Read the model definition and answer for the solid it produces. Units are mm, in the model's axes. A direction names the side the tool comes from. Coordinates: 2 decimals unless noted, no trailing zeros. Loops run counter-clockwise (first coordinate to the right, second up) from the corner with the lowest first, then second, coordinate; pieces in that order, holes last. Notation, with made-up numbers: M 75,34 L 123,34 A28 cw 123,56 Z; hole C 81.25,-26.5 d5. An arc over 180 degrees is marked long. One line per item, written item: value. Start each with the question number.
```python
from build123d import *

# Parameters (mm, degrees)
F0_W     = 91.7135253549
F0_H     = 27.9620755464
F1_DEPTH = 3.175
F4_W     = 2.665694803
F4_H     = 11.1176939681
F5_DEPTH = 10.16
F7_W     = 36.2722687423
F7_H     = 13.592146337
F8_DEPTH = 68.072


with BuildPart() as f1:
    # F0 (on Top) → F1 (new body)
    with BuildSketch(Plane.XY):
        Rectangle(F0_W, F0_H)
    extrude(amount=F1_DEPTH)

    # F4 (on line) → F5 (join)
    with BuildSketch(Plane(origin=(0, 0, 0), x_dir=(1, 0, 0), z_dir=(0, 0.3420201433, 0.9396926208))):
        with Locations((16.3055844605, 0)):
            Rectangle(F4_W, F4_H)
    extrude(amount=F5_DEPTH)

    # F6: F1 across plane


with BuildPart() as f1_1:
    add(f1.part)
    add(f1.part.mirror(Plane.YZ))

    # F7 (on Right) → F8 (cut, symmetric)
    with BuildSketch(Plane.YZ):
        with Locations((0.2234503627, -6.7960731685)):
            Rectangle(F7_W, F7_H)
    extrude(amount=F8_DEPTH, both=True, mode=Mode.SUBTRACT)


solid = f1_1.part
```
1) Section B-B (y = -3) is taken. Determine the outline of the cut face in (x, z) (3 decimals), then the cut area to 3 significant figures.
2) Consider line 1 along X through (y, z) = (7.25, 7); line 2 along Z through (x, y) = (11, 9.75) (3 decimals). Determine where each line is inside the solid, lowest interval first.
3) Section D-D (z = 4.75) is taken. Determine the outline of the cut face in (x, y), then the cut area to 3 significant figures.
4) Section A-A (z = 10) is taken. Determine the outline of the cut face in (x, y).
5) Flat-ended cylindrical pins translate along their axes: pin 1 (1 mm diameter, centred on y = -3.5, z = 9.5, fed in from +X); pin 2 (3 mm diameter, centred on x = -2, y = 6, fed in from -Z); pin 3 (10 mm diameter, centred on x = 18, y = -11, fed in from +Z) (3 decimals); pin 4 (2.5 mm diameter, centred on y = 3.5, z = 5.5, fed in from +X). Find the tip coordinate at first contact, or state that the pin passes through.
6) Section C-C (x = 11.5) is taken. Determine the outline of the cut face in (y, z) (3 decimals).
7) A tool of negligible diameter and unlimited length cuts with its end or side. For faces 4 (the face through (-14.973, 2, 6)), 5 (the face through (-16.287, 7.873, 5.379)), 6 (the face through (-17.638, 2, 6)), from which of +Z, -Z, +X, -X, +Y, -Y can it reach the whole face along a straight path? Write none if from no direction.
8) For a pull along X with two mould halves and no side action, classify faces 1 (the face through (-1, 0, 3.175)), 2 (the face through (16.287, 7.873, 5.379)), 3 (the face through (-45.857, 0, 2)) as released by +X, released by -X, zero draft, split by the parting line, or undercut.
Results found:
1. outline: M -45.857,0 L 45.857,0 L 45.857,3.175 L 17.638,3.175 L 17.638,8.011 L 14.973,8.011 L 14.973,3.175 L -14.973,3.175 L -14.973,8.011 L -17.638,8.011 L -17.638,3.175 L -45.857,3.175 Z
1. area: 317 mm²
2. line 1: x = -17.64 to -14.97, 14.97 to 17.64
2. line 2: z = 0 to 3.175
3. outline: M -17.64,-4.19 L -14.97,-4.19 L -14.97,7.64 L -17.64,7.64 Z; M 14.97,-4.19 L 17.64,-4.19 L 17.64,7.64 L 14.97,7.64 Z
3. area: 63.1 mm²
4. outline: M -17.64,-2.28 L -14.97,-2.28 L -14.97,2.23 L -17.64,2.23 Z; M 14.97,-2.28 L 17.64,-2.28 L 17.64,2.23 L 14.97,2.23 Z
5. pin 1: passes through
5. pin 2: stops at z = 0
5. pin 3: stops at z = 3.175
5. pin 4: stops at x = 17.64
6. outline: M -13.981,0 L 13.981,0 L 13.981,3.175 L -13.981,3.175 Z
7. face 4: +Z, +Y, -Y
7. face 5: +X, -X, +Y
7. face 6: +Z, -X, +Y, -Y
8. face 1: undercut
8. face 2: zero draft
8. face 3: released by -X
